```python
from build123d import *

# Parameters (mm, degrees)
F0_W      = 42
F0_H      = 42
F1_DEPTH  = 33
F2_R      = 11
F3_DEPTH  = 2
F4_R      = 2.5
F5_DEPTH  = 20
F6_R      = 1.5
F7_DEPTH  = 4.5
F8_SIZE   = 5
F9_R      = 4
F10_R     = 1.5
F11_DEPTH = 25


with BuildPart() as f1:
    # F0 (on Top) → F1 (new body)
    with BuildSketch(Plane.XY):
        with Locations((21, -21)):
            Rectangle(F0_W, F0_H)
    extrude(amount=F1_DEPTH)

    # F2 (on face) → F3 (join)
    with BuildSketch(Plane.XY.offset(33)):
        with Locations((21, -21)):
            Circle(F2_R)
    extrude(amount=F3_DEPTH)

    # F4 (on face) → F5 (join)
    with BuildSketch(Plane.XY.offset(35)):
        with Locations((21, -21)):
            Circle(F4_R)
    extrude(amount=F5_DEPTH)

    # F6 (on face) → F7 (cut)
    with BuildSketch(Plane.XY.offset(33)):
        with Locations((5.5, -5.5)):
            Circle(F6_R)
        with Locations((36.5, -5.5)):
            Circle(F6_R)
        with Locations((36.5, -36.5)):
            Circle(F6_R)
        with Locations((5.5, -36.5)):
            Circle(F6_R)
    extrude(amount=-F7_DEPTH, mode=Mode.SUBTRACT)

    # F8
    f8_edges = [f1.edges().sort_by_distance(p)[0] for p in [
        (42, 0, 16.5),
        (42, -42, 16.5),
        (0, -42, 16.5),
        (0, 0, 16.5),
    ]]
    chamfer(f8_edges, length=F8_SIZE)

    # F9
    f9_edges = [f1.edges().sort_by_distance(p)[0] for p in [
        (0, -5, 16.5),
        (5, 0, 16.5),
        (0, -37, 16.5),
        (5, -42, 16.5),
        (37, -42, 16.5),
        (42, -37, 16.5),
        (37, 0, 16.5),
        (42, -5, 16.5),
    ]]
    fillet(f9_edges, radius=F9_R)

    # F10 (on face) → F11 (cut)
    with BuildSketch(Plane(origin=(0, 0, 0), x_dir=(1, 0, 0), z_dir=(0, 0, -1))):
        with Locations((36.5, 36.5)):
            Circle(F10_R)
        with Locations((5.5, 36.5)):
            Circle(F10_R)
        with Locations((5.5, 5.5)):
            Circle(F10_R)
        with Locations((36.5, 5.5)):
            Circle(F10_R)
    extrude(amount=-F11_DEPTH, mode=Mode.SUBTRACT)


solid = f1.part
```
For this review, take the finished solid that the model builds, in its own axes (mm). A direction names the side the tool comes from. Coordinates: 2 decimals unless noted, no trailing zeros. Order: outer loops, then holes, each group sorted by start corner. A loop starts at its lowest first (then second) coordinate and runs counter-clockwise, first axis right, second up. Notation, with made-up numbers: (18, 32) -> (23, 32) arc R21 ccw to (23, 70) -> close; hole circle Ø5 at (22, -2.75). An arc over 180 degrees is marked (long way). Use CSV: the item, a comma, the result in double quotes. Start each with the question number.
Item 1: We need section C-C, the plane x = 21. Give the boundary of the cut face in (y, z).
Item 2: Insertion check: pin 1 (3.5 mm diameter, centred on x = 5, y = -36.5, fed in from +Z); pin 2 (0.9 mm diameter, centred on x = 37, y = -36.5, fed in from +Z); pin 3 (1.8 mm diameter, centred on x = 5.5, y = -36.5, fed in from -Z). Each pin has a flat end and moves straight along its axis. Give the tip position at first contact, or say it passes through.
Item 3: For faces 4 (the face through (5.175, -35.036, 12.325)), 5 (the face through (21, -21, 55)), 6 (the face through (35.3, -6.4, 30.8)), list the 3-axis set-ups (+Z, -Z, +X, -X, +Y, -Y) from which the entire face can be reached by the end or side of a thin tool; tool diameter is ignored.
Item 4: Draft analysis for pull direction X (two halves, no side actions). For faces 1 (the face through (5.11, -41.69, 16.73)), 2 (the face through (5, -37, 25)), 3 (the face through (30, -30, 33)), state which applies: pulls with the +X half, pulls with the -X half, needs draft (parallel to the pull), parting line crosses it, or undercut.
Item 5: Wall thickness on probe 1 along Y at (x, z) = (36.5, 12.25); probe 2 along X at (y, z) = (-36.5, 6.25); probe 3 along Y at (x, z) = (5, 31): over which ranges is each line inside the solid? List them lowest first.
Item 6: We need section A-A, the plane z = 10. Give the boundary of the cut face in (x, y), then the cut area to 3 significant figures.
Item 7: We need section B-B, the plane y = -21. Give the boundary of the cut face in (x, z).
Item 8: We need section D-D, the plane z = 26. Give the boundary of the cut face in (x, y).
Derived:
1,outline,"(-42, 0) -> (0, 0) -> (0, 33) -> (-10, 33) -> (-10, 35) -> (-18.5, 35) -> (-18.5, 55) -> (-23.5, 55) -> (-23.5, 35) -> (-32, 35) -> (-32, 33) -> (-42, 33) -> close"
2,pin 1,"stops at z = 33"
2,pin 2,"stops at z = 28.5"
2,pin 3,"stops at z = 25"
3,face 4,"-Z"
3,face 5,"+Z, +X, -X, +Y, -Y"
3,face 6,"+Z"
4,face 1,"pulls with the -X half"
4,face 2,"undercut"
4,face 3,"needs draft"
5,probe 1,"y = -41.83 to -38, -35 to -7, -4 to -0.17"
5,probe 2,"x = 0.17 to 4, 7 to 35, 38 to 41.83"
5,probe 3,"y = -41.64 to -37.91, -35.09 to -6.91, -4.09 to -0.36"
6,outline,"(0, -35.34) arc R4 ccw to (1.17, -38.17) -> (3.83, -40.83) arc R4 ccw to (6.66, -42) -> (35.34, -42) arc R4 ccw to (38.17, -40.83) -> (40.83, -38.17) arc R4 ccw to (42, -35.34) -> (42, -6.66) arc R4 ccw to (40.83, -3.83) -> (38.17, -1.17) arc R4 ccw to (35.34, 0) -> (6.66, 0) arc R4 ccw to (3.83, -1.17) -> (1.17, -3.83) arc R4 ccw to (0, -6.66) -> close; hole circle Ø3 at (5.5, -36.5); hole circle Ø3 at (5.5, -5.5); hole circle Ø3 at (36.5, -36.5); hole circle Ø3 at (36.5, -5.5)"
6,area,"1,680 mm^2"
7,outline,"(0, 0) -> (42, 0) -> (42, 33) -> (32, 33) -> (32, 35) -> (23.5, 35) -> (23.5, 55) -> (18.5, 55) -> (18.5, 35) -> (10, 35) -> (10, 33) -> (0, 33) -> close"
8,outline,"(0, -35.34) arc R4 ccw to (1.17, -38.17) -> (3.83, -40.83) arc R4 ccw to (6.66, -42) -> (35.34, -42) arc R4 ccw to (38.17, -40.83) -> (40.83, -38.17) arc R4 ccw to (42, -35.34) -> (42, -6.66) arc R4 ccw to (40.83, -3.83) -> (38.17, -1.17) arc R4 ccw to (35.34, 0) -> (6.66, 0) arc R4 ccw to (3.83, -1.17) -> (1.17, -3.83) arc R4 ccw to (0, -6.66) -> close"
